Could you check a few things on this drawing? It's one solid part, dimensions in mm from its lowest x, y, z. Round coordinates to 2 decimals unless told otherwise and drop trailing zeros. Order: outer loops, then holes, each group sorted by start corner. A loop starts at its lowest first (then second) coordinate and runs counter-clockwise, first axis right, second up. Notation, with made-up numbers: M -15.5,61 L 0.5,61 A22 cw 0.5,99 Z; hole C 37,3.25 d8. An arc over 180 degrees is marked long. Answer as a JSON object with one key per item and string values. Group by question number.
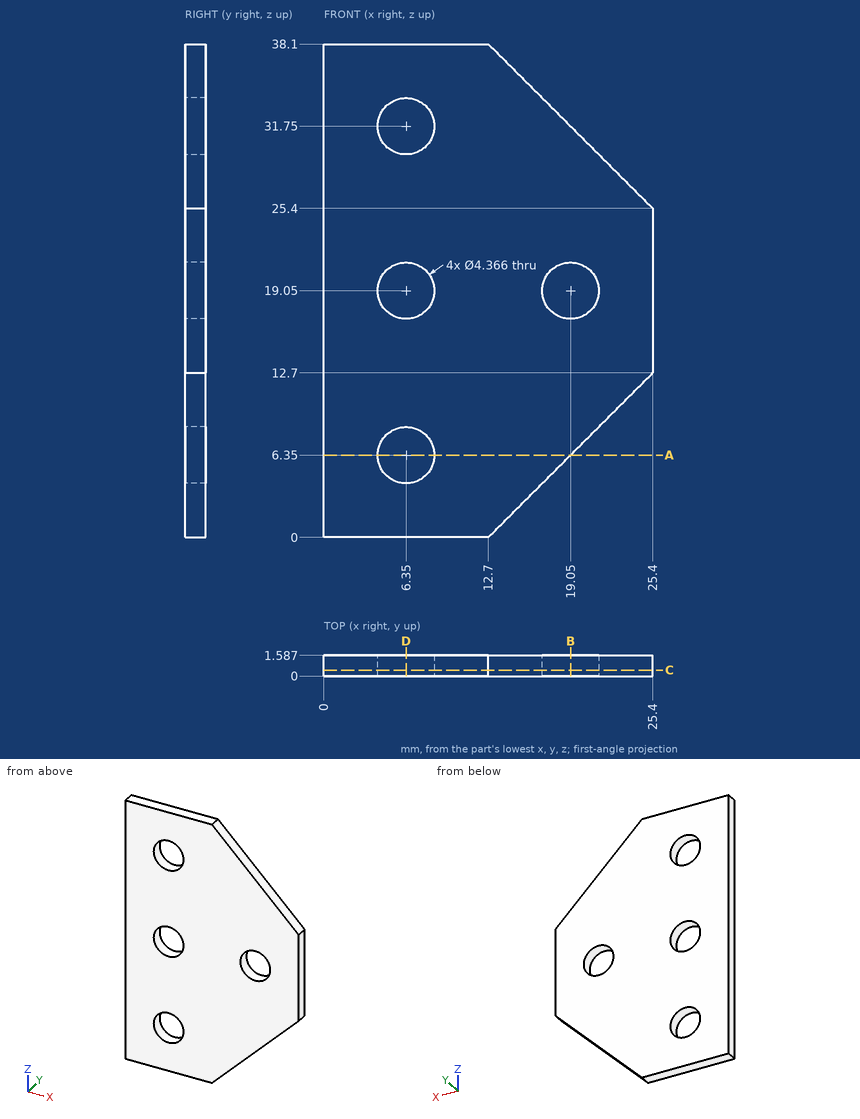
1) If we section it at A-A on z = 6.35: Write out the boundary of the cut face in (x, y).
2) If we section it at C-C on y = 0.45: Count the separate pieces of the cut face and the enclosed holes in it.
3) I need wall thicknesses on line 1 along Z through (x, y) = (6.35, 1); line 2 along Z through (x, y) = (8.25, 0.95) (1 decimal); line 3 along X through (y, z) = (0.85, 21) (1 decimal). Which ranges of each line are inside material? Lowest first, please.
4) If we section it at D-D on x = 6.35: Write out the boundary of the cut face in (y, z).
5) If we section it at B-B on x = 19.05: Write out the boundary of the cut face in (y, z).
Findings:
{
 "1": {"outline": "M 0,0 L 4.17,0 L 4.17,1.59 L 0,1.59 Z; M 8.53,0 L 19.05,0 L 19.05,1.59 L 8.53,1.59 Z"},
 "2": {"separate pieces": "1", "enclosed holes": "4"},
 "3": {"line 1": "z = 0 to 4.17, 8.53 to 16.87, 21.23 to 29.57, 33.93 to 38.1", "line 2": "z = 0 to 5.3, 7.4 to 18, 20.1 to 30.7, 32.8 to 38.1", "line 3": "x = 0 to 5.4, 7.3 to 18.1, 20 to 25.4"},
 "4": {"outline": "M 0,0 L 1.59,0 L 1.59,4.17 L 0,4.17 Z; M 0,8.53 L 1.59,8.53 L 1.59,16.87 L 0,16.87 Z; M 0,21.23 L 1.59,21.23 L 1.59,29.57 L 0,29.57 Z; M 0,33.93 L 1.59,33.93 L 1.59,38.1 L 0,38.1 Z"},
 "5": {"outline": "M 0,6.35 L 1.59,6.35 L 1.59,16.87 L 0,16.87 Z; M 0,21.23 L 1.59,21.23 L 1.59,31.75 L 0,31.75 Z"}
}
